Design review of the part built by this model. Coordinates are the model's own, in mm. A direction names the side the tool comes from. Round coordinates to 2 decimals unless told otherwise and drop trailing zeros. Loops run counter-clockwise (first coordinate to the right, second up) from the corner with the lowest first, then second, coordinate; pieces in that order, holes last. Notation, with made-up numbers: (-6, -31.5) - (41, -31.5) arc R9 ccw to (41, -23.5) - close; hole circle Ø7 at (-12, -33.5). An arc over 180 degrees is marked (long way). Use one line per item in the form item = value. Start each with the question number.
(1) We need section D-D, the plane y = 34. Write out the cut boundary in (x, z), then the cut area to 3 significant figures.
(2) The part is to be moulded in two halves that separate along X. For faces 1 (the cylindrical face through (0, 18, 0.5)), 2 (the cylindrical face through (-0.217, 19.024, 0.493)), 3 (the flat face through (0, 42, 3)), say which applies: released by +X, released by -X, zero draft, split by the parting line, or undercut.
(3) We need section B-B, the plane y = 48.5. Write out the cut boundary in (x, z), then the cut area to 3 significant figures.
(4) Wall thickness on probe 1 along Y at (x, z) = (0, 0.5); probe 2 along X at (y, z) = (20, 0.25); probe 3 along Z at (x, y) = (-1.5, 21.5): over which ranges is each line inside the solid? List them lowest first. Write a range as [from, to].
(5) For pin 1 (1 mm diameter, centred on y = 39.5, z = 1, fed in from +X); pin 2 (1.5 mm diameter, centred on x = -1.5, z = 1, fed in from +Y); pin 3 (2.5 mm diameter, centred on x = -0.5, y = 22.5, fed in from +Z), all flat-tipped, find the tip position at first contact; note any pin that passes through.
(6) We need section C-C, the plane z = 1.35. Write out the cut boundary in (x, y).
(7) We need section A-A, the plane x = 0. Write out the cut boundary in (y, z), then the cut area to 3 significant figures.
(8) Machinability: for faces 4 (the flat face through (3.2, 37.9, 1.5)), 5 (the cylindrical face through (0, 30, 2)), which of the approach directions +Z, -Z, +X, -X, +Y, -Y give a long, thin tool a straight path to every point of the face, cutting with its end or side? Answer none if there is none.
from build123d import *

# Parameters (mm, degrees)
SKETCH1_R           = 2
SKETCH1_R_2         = 1
BOSS_EXTRUDE1_DEPTH = 3
SKETCH2_R           = 10
CUT_EXTRUDE1_DEPTH  = 2


with BuildPart() as part:
    # Sketch1 → Boss-Extrude1 (new body)
    with BuildSketch(Plane.XY):
        with BuildLine():
            Line((1.995550606, 19.866666667), (3.991101213, 49.733333333))
            ThreePointArc((3.991101213, 49.733333333), (0, 54), (-3.991101213, 49.733333333))
            Line((-3.991101213, 49.733333333), (-1.995550606, 19.866666667))
            ThreePointArc((-1.995550606, 19.866666667), (0, 18), (1.995550606, 19.866666667))
        make_face()
        with Locations((0, 50)):
            Circle(SKETCH1_R, mode=Mode.SUBTRACT)
        with Locations((0, 20)):
            Circle(SKETCH1_R_2, mode=Mode.SUBTRACT)
    extrude(amount=BOSS_EXTRUDE1_DEPTH)

    # Sketch2 → Cut-Extrude1 (cut)
    with BuildSketch(Plane.XY.offset(3)):
        with Locations((0, 20)):
            Circle(SKETCH2_R)
    extrude(amount=-CUT_EXTRUDE1_DEPTH, mode=Mode.SUBTRACT)


solid = part.part
Data:
q1.outline = (-2.94, 0) - (2.94, 0) - (2.94, 3) - (-2.94, 3) - close
q1.area = 17.6 mm^2
q2.face_1 = split by the parting line
q2.face_2 = undercut
q2.face_3 = zero draft
q3.outline = (-3.91, 0) - (-1.32, 0) - (-1.32, 3) - (-3.91, 3) - close; (1.32, 0) - (3.91, 0) - (3.91, 3) - (1.32, 3) - close
q3.area = 15.5 mm^2
q4.probe_1 = [18, 19], [21, 48], [52, 54]
q4.probe_2 = [-2, -1], [1, 2]
q4.probe_3 = [0, 1]
q5.pin_1 = 3.34
q5.pin_2 = 53.93
q5.pin_3 = 1
q6.outline = (-3.99, 49.73) - (-2.65, 29.64) arc R10 cw to (2.65, 29.64) - (3.99, 49.73) arc R4 ccw (long way) to start; hole circle Ø4 at (0, 50)
q7.outline = (18, 0) - (19, 0) - (19, 1) - (18, 1) - close; (21, 0) - (48, 0) - (48, 3) - (30, 3) - (30, 1) - (21, 1) - close; (52, 0) - (54, 0) - (54, 3) - (52, 3) - close
q7.area = 70.0 mm^2
q8.face_4 = +Z, -Z, +X, -Y
q8.face_5 = +Z, -Y
